from build123d import *

# Parameters (mm, degrees)
SKETCH033_R             = 3
PAD015_DEPTH            = 4
SKETCH035_W             = 0.6
SKETCH035_H             = 4
POCKET014_DEPTH         = 8.552756
SKETCH008_R             = 2.6
PAD016_DEPTH            = 4
SKETCH034_R             = 8
PAD017_DEPTH            = 3
CHAMFER010_SIZE         = 1
BODY005_PLACEMENT_ANGLE = 135


with BuildPart() as part:
    # Sketch032 → Revolution (revolve)
    with BuildSketch(Plane.XZ):
        with BuildLine():
            Line((-2.2, 0), (-2.2, -2))
            Line((-2.2, -2), (-2.2, -5))
            Line((-2.2, -5), (-2.8, -5))
            Line((-2.8, -5), (-4.923191, -2.876809))
            ThreePointArc((-4.923191, -2.876809), (-8.269417, -5.211047), (-10.611545, -8.551756))
            Line((-10.611545, -8.551756), (-10.974068, -8.382708))
            ThreePointArc((-8.562033, -4.937967), (-9.918738, -6.554825), (-10.974068, -8.382708))
            Line((-8.562033, -4.937967), (-2.6, 1.024067))
            Line((-2.6, 1.024067), (-2.6, 0))
            Line((-2.6, 0), (-2.2, 0))
        make_face()
    revolve(axis=Axis((0, 0, 0), (0, 0, 1)))

    # Sketch033 → Pad015 (new body)
    with BuildSketch(Plane.XY):
        Circle(SKETCH033_R)
        with BuildLine():
            Line((1.609348, 1.5), (-1.609348, 1.5))
            ThreePointArc((-1.609348, 1.5), (-2.2, 0), (-1.609348, -1.5))
            Line((-1.609348, -1.5), (1.609348, -1.5))
            ThreePointArc((1.609348, -1.5), (2.2, 0), (1.609348, 1.5))
        make_face(mode=Mode.SUBTRACT)
    extrude(amount=-PAD015_DEPTH)

    # Sketch035 → Pocket014 (cut, through all)
    with BuildSketch(Plane.XY):
        Rectangle(SKETCH035_W, SKETCH035_H)
    extrude(amount=-POCKET014_DEPTH, mode=Mode.SUBTRACT)

    # Sketch008 → Pad016 (join)
    with BuildSketch(Plane.XY):
        Circle(SKETCH008_R)
    extrude(amount=PAD016_DEPTH)

    # Sketch034 (on Face4 of Pad016) → Pad017 (join)
    with BuildSketch(Plane(origin=(0, 0, 4), x_dir=(-1, 0, 0), z_dir=(0, 0, 1))):
        Circle(SKETCH034_R)
    extrude(amount=PAD017_DEPTH)

    # Chamfer010
    chamfer010_edges = [part.edges().sort_by_distance(p)[0] for p in [
        (8, 0, 7),
    ]]
    chamfer(chamfer010_edges, length=CHAMFER010_SIZE)


with BuildPart() as part_1:
    # Body005 placement: moved
    add(part.part.moved(Location((128.68, -199, 22))).rotate(Axis((128.68, -199, 22), (0, 0, 1)), BODY005_PLACEMENT_ANGLE))


solid = part_1.part
Geometry: final body of the model. Coordinates: model frame, mm. A direction names the side the tool comes from. Round coordinates to 2 decimals unless told otherwise and drop trailing zeros. Loops run counter-clockwise (first coordinate to the right, second up) from the corner with the lowest first, then second, coordinate; pieces in that order, holes last.
Q1. Pin query (flat end, axial travel): P1, Ø6, axis at y = -199, z = 16, coming from the +X side; P2, Ø13, axis at x = 128.5, y = -201, coming from the -Z side; P3, Ø6, axis at x = 120, z = 26.5, coming from the -Y side; P4, Ø6, axis at y = -204, z = 23.5, coming from the +X side. Return the tip coordinate at first contact, or that it passes through.
Q2. Section A-A on z = 19.5. Return loops of the section in (x, y), plus the area to 3 significant figures.
Q3. Section C-C on z = 24. Return loops of the section in (x, y).
Q4. Access query for faces 1 (the cylindrical face through (120.75, -197.95, 26.99)), 2 (the conical face through (128.55, -196.11, 22.73)), 3 (the flat face through (127, -200, 18)). Directions: +Z, -Z, +X, -X, +Y, -Y. A direction counts if a zero-diameter tool reaches every point of the face in a straight line with its end or side. Return the directions, or none.
Q5. Material intervals for L1, parallel to Y at x = 128.68, z = 18.2; L2, parallel to Y at x = 128.68, z = 18.6; L3, parallel to Y at x = 128.68, z = 20.75, sorted ascending.
Q6. Pull-direction query (X, two-part tool) for faces 4 (the flat face through (129, -199, 29)), 5 (the flat face through (129, -199, 22)), 6 (the cylindrical face through (126.374, -197.799, 24.491)); classes: released by +X, released by -X, zero draft, split by the parting line, or undercut.
Q7. Section B-B on z = 27. Return loops of the section in (x, y), plus the area to 3 significant figures.
Evaluation:
1. P1: stops at x = 139.65
1. P2: stops at z = 16.54
1. P3: stops at y = -204.63
1. P4: stops at x = 135.95
2. outline: circle Ø12.25 at (128.68, -199); hole (126.48, -198.92) - (127.41, -199.85) - (127.05, -200.2) - (127.48, -200.63) - (127.83, -200.27) - (128.76, -201.2) arc R2.2 ccw to (130.88, -199.08) - (129.95, -198.15) - (130.31, -197.8) - (129.88, -197.37) - (129.53, -197.73) - (128.6, -196.8) arc R2.2 ccw to start
2. area: 105 mm2
3. outline: circle Ø5.2 at (128.68, -199)
4. face 1: +Z
4. face 2: none
4. face 3: -Z
5. L1: y = -206.42 to -205.56, -203 to -201.12, -196.88 to -195, -192.44 to -191.58
5. L2: y = -206.02 to -204.92, -203.4 to -201.12, -196.88 to -194.6, -193.08 to -191.98
5. L3: y = -203.87 to -201.12, -196.88 to -194.13
6. face 4: zero draft
6. face 5: undercut
6. face 6: split by the parting line
7. outline: circle Ø16 at (128.68, -199)
7. area: 201 mm2
